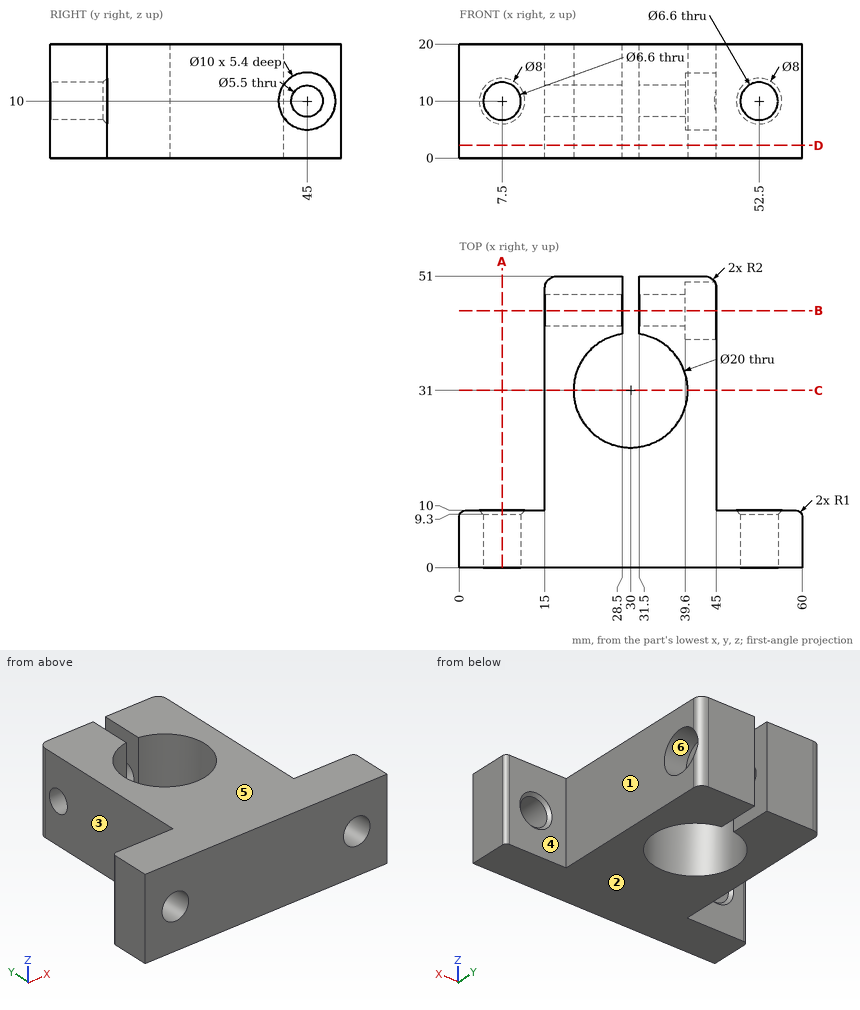
Geometry check sheet. Reference: drawing and pictorial views, mm from the part's lowest x, y, z. A direction names the side the tool comes from. Coordinates: 2 decimals unless noted, no trailing zeros. Write each loop counter-clockwise with the first axis right and the second up, starting at its lowest first coordinate (ties: lowest second). Pieces come first, ordered by that corner, then holes. Notation, with made-up numbers: (27, 29) - (52, 29) arc R23 cw to (52, 41) - close; hole circle Ø11 at (37, -12.5). An arc over 180 degrees is marked (long way). Write item = value, one per line.
Q1. Go/stop test with flat-tipped pins: pin 1 Ø6 at (x, z) = (7.5, 10) entering from +Y; pin 2 Ø8 at (y, z) = (43.5, 9) entering from +X; pin 3 Ø9 at (y, z) = (45, 10) entering from +X; pin 4 Ø7 at (x, z) = (54.5, 11.5) entering from +Y. Record where each tip stops, or that it passes through.
Answer:
pin_1 = through
pin_2 = 45
pin_3 = 39.6
pin_4 = 10
Q2. Mould release check, pull along Z, two halves, no side actions. Record for the marked faces 4, 5 and 6: released by +Z, released by -Z, zero draft, split by the parting line, or undercut.
Answer:
face_4 = zero draft
face_5 = released by +Z
face_6 = undercut
Q3. Access from +Z, -Z, +X, -X, +Y, -Y to the whole of each face (thin tool, end or side, straight path). Record for the marked faces 1, 2 and 3.
Answer:
face_1 = +Z, -Z, +X, +Y
face_2 = -Z, +X, -X, +Y, -Y
face_3 = +Z, -Z, -X, +Y
Q4. Material ranges on L1, parallel to Y at x = 28, z = 11.5; L2, parallel to Z at x = 35, y = 45; L3, parallel to Z at x = 40.5, y = 45, recorded low to high. Write a range as from..to.
Answer:
L1 = 0..21.2, 40.8..42.7, 47.3..51
L2 = 0..7.25, 12.75..20
L3 = 0..5, 15..20
Q5. Cross-section at D-D (z = 2.25). Enter the section's corners in (x, y), plus the area to 3 significant figures.
Answer:
outline = (0, 0) - (60, 0) - (60, 9) arc R1 ccw to (59, 10) - (45, 10) - (45, 49) arc R2 ccw to (43, 51) - (31.5, 51) - (31.5, 40.89) arc R10 cw (long way) to (28.5, 40.89) - (28.5, 51) - (17, 51) arc R2 ccw to (15, 49) - (15, 10) - (1, 10) arc R1 ccw to (0, 9) - close
area = 1,480 mm²
Q6. Cross-section at C-C (y = 31). Enter the section's corners in (x, z), plus the area to 3 significant figures.
Answer:
outline = (15, 0) - (20, 0) - (20, 20) - (15, 20) - close; (40, 0) - (45, 0) - (45, 20) - (40, 20) - close
area = 200 mm²
Q7. Cross-section at A-A (x = 7.5). Enter the section's corners in (y, z).
Answer:
outline = (0, 0) - (10, 0) - (10, 6) - (9.3, 6.7) - (0, 6.7) - close; (0, 13.3) - (9.3, 13.3) - (10, 14) - (10, 20) - (0, 20) - close
Q8. Cross-section at B-B (y = 45). Enter the section's corners in (x, z).
Answer:
outline = (15, 0) - (28.5, 0) - (28.5, 7.25) - (15, 7.25) - close; (15, 12.75) - (28.5, 12.75) - (28.5, 20) - (15, 20) - close; (31.5, 0) - (45, 0) - (45, 5) - (39.6, 5) - (39.6, 7.25) - (31.5, 7.25) - close; (31.5, 12.75) - (39.6, 12.75) - (39.6, 15) - (45, 15) - (45, 20) - (31.5, 20) - close
